Here's the drawing with two shaded views (mm, measured from the low corner). I have some questions. A direction names the side the tool comes from. Give positions to 0.01 mm unless a question says otherwise; leave off trailing zeros. Loops run counter-clockwise (first coordinate to the right, second up) from the corner with the lowest first, then second, coordinate; pieces in that order, holes last. Notation, with made-up numbers: M 84,5.5 L 128,5.5 A8 cw 128,10.5 Z; hole C 33.5,18 d3. An arc over 180 degrees is marked long. Use a Markdown table: item, result. Add a question column.
1) Suppose I cut it at A-A on x = 47.5. List the corners of the cut face in (y, z) for me.
2) Will these pins go through, and if not, where does the flat tip stop? pin 1 Ø4 at (y, z) = (326.5, 56.5) entering from +X; pin 2 Ø1.5 at (y, z) = (196, 18) entering from +X; pin 3 Ø8 at (y, z) = (171, 64) entering from -X.
3) Suppose I cut it at D-D on z = 116.5. List the corners of the cut face in (x, y) for me.
4) Which directions (+Z, -Z, +X, -X, +Y, -Y) give clear straight access to the entire face, cutting with the end or side of a thin tool? Please do the marked faces 4 and 5.
5) Suppose I cut it at B-B on y = 58. List the corners of the cut face in (x, z) for me, and give its area (3 significant figures).
6) We'd pull the mould along Z, two halves only. Please class the marked faces 1, 2 and 3: +Z half, -Z half, draft (parallel to the pull), parting line (faces both ways), or undercut.
7) If I drill on line 1 along Z through (x, y) = (59, 376.5); line 2 along X through (y, z) = (105.5, 92); line 3 along Z through (x, y) = (96.5, 289), over which ranges is the centre line in solid material (lowest first)? Write a range as [from, to].
8) Suppose I cut it at C-C on x = 68.5. List the corners of the cut face in (y, z) for me.
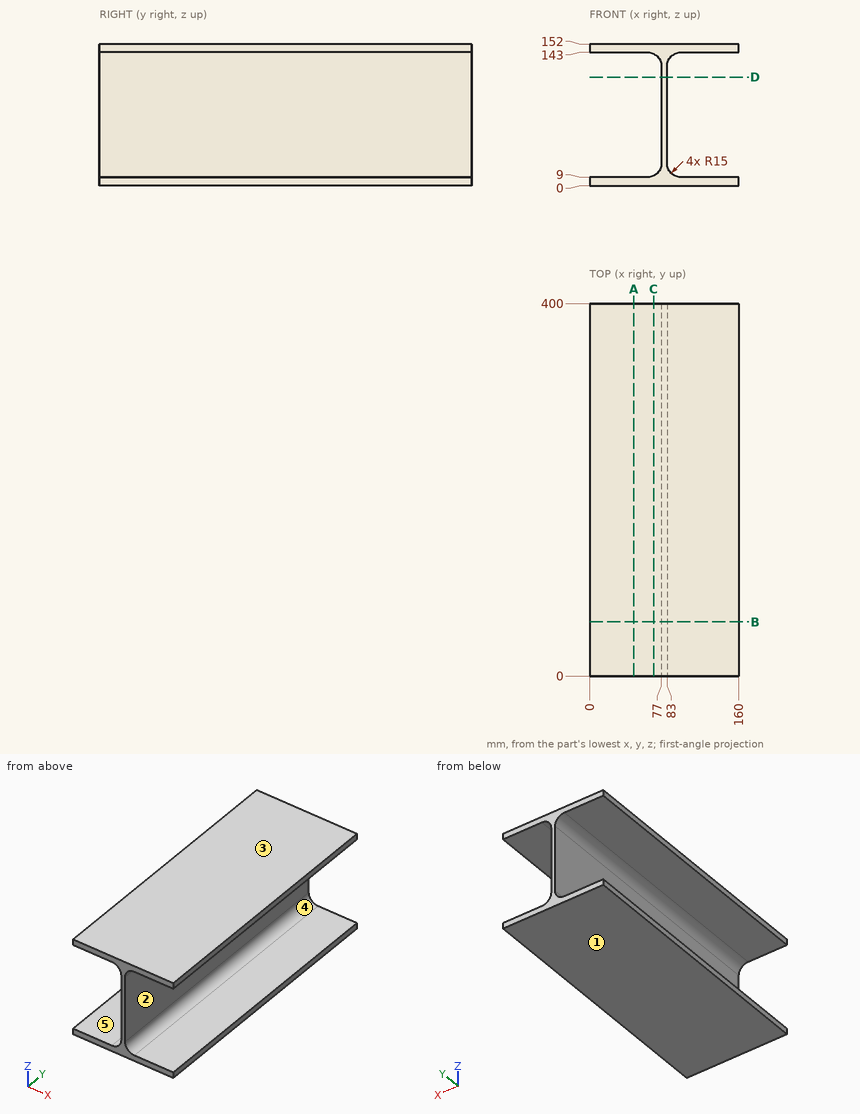
Answer block:
| question | item | result |
|---|---|---|
| 1 | outline | M 0,0 L 400,0 L 400,9 L 0,9 Z; M 0,143 L 400,143 L 400,152 L 0,152 Z |
| 2 | pin 1 | stops at x = 83 |
| 2 | pin 2 | stops at x = 84.6 |
| 2 | pin 3 | stops at x = 77 |
| 3 | outline | M 77,0 L 83,0 L 83,400 L 77,400 Z |
| 4 | face 4 | +X, +Y, -Y |
| 4 | face 5 | -X, +Y, -Y |
| 5 | outline | M 0,0 L 160,0 L 160,9 L 98,9 A15 cw 83,24 L 83,128 A15 cw 98,143 L 160,143 L 160,152 L 0,152 L 0,143 L 62,143 A15 cw 77,128 L 77,24 A15 cw 62,9 L 0,9 Z |
| 5 | area | 3,880 mm^2 |
| 6 | face 1 | -Z half |
| 6 | face 2 | undercut |
| 6 | face 3 | +Z half |
| 7 | line 1 | z = [0, 9], [143, 152] |
| 7 | line 2 | x = [77, 83] |
| 7 | line 3 | z = [0, 9.08], [142.92, 152] |
| 8 | outline | M 0,0 L 400,0 L 400,10.48 L 0,10.48 Z; M 0,141.52 L 400,141.52 L 400,152 L 0,152 Z |
